For this review, take the finished solid that the model builds, in its own axes (mm). Face numbers are marked on the shaded views. A direction names the side the tool comes from. Round coordinates to 2 decimals unless told otherwise and drop trailing zeros. Loops run counter-clockwise (first coordinate to the right, second up) from the corner with the lowest first, then second, coordinate; pieces in that order, holes last.
1) Wall thickness on L1, parallel to Y at x = -10, z = 2.25; L2, parallel to X at y = 10, z = 3.45; L3, parallel to Z at x = 4.25, y = 9.5: over which ranges is each line inside the solid? List them lowest first.
2) Insertion check: pin 1 (4 mm diameter, centred on x = 6.5, y = 10, fed in from +Z); pin 2 (1 mm diameter, centred on x = 4.5, z = 19, fed in from -Y). Each pin has a flat end and moves straight along its axis. Give the tip position at first contact, or say it passes through.
3) Take a section at D-D (z = 3.5). State the section outline as (x, y) points, then the cut area to 3 significant figures.
4) Take a section at B-B (x = -10). State the section outline as (y, z) points.
5) Tool access review of the marked faces 1 and 2: name each direction out of +Z, -Z, +X, -X, +Y, -Y from which nothing blocks a thin tool from reaching the whole face with its end or side.
6) Take a section at A-A (z = 35). State the section outline as (x, y) points, then the cut area to 3 significant figures.
7) Take a section at C-C (y = -10). State the section outline as (x, z) points.
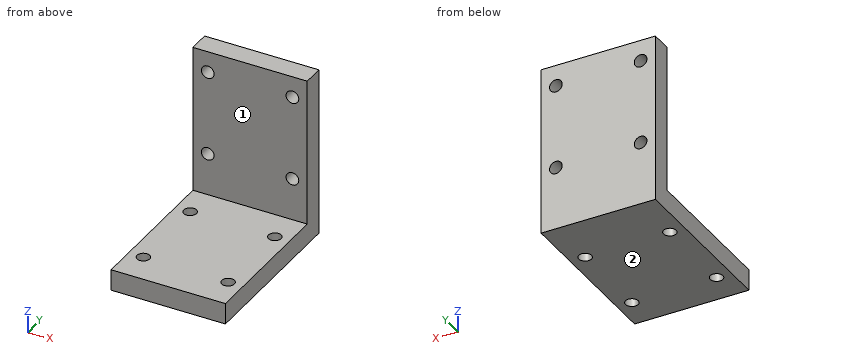
```python
from build123d import *

# Parameters (mm, degrees)
F0_W      = 27
F0_H      = 35
F1_DEPTH  = 5
F2_D      = 3
F1_FACE_W = 27
F1_FACE_H = 5
F3_DEPTH  = 5
F4_W      = 5
F4_H      = 40
F5_DEPTH  = 13.5
F7_D      = 3


with BuildPart() as f1:
    # F0 (on Top) → F1 (new body)
    with BuildSketch(Plane.XY):
        Rectangle(F0_W, F0_H)
    extrude(amount=F1_DEPTH)

    # F2 (through all)
    with Locations(Plane(origin=(0, 0, 0), x_dir=(1, 0, 0), z_dir=(0, 0, -1))):
        with Locations((-10, 10), (10, 10), (10, -10), (-10, -10)):
            Hole(F2_D / 2)

    # F1_face (on face) → F3 (join)
    with BuildSketch(Plane(origin=(0, 17.5, 2.5), x_dir=(-1, 0, 0), z_dir=(0, 1, 0))):
        Rectangle(F1_FACE_W, F1_FACE_H)
    extrude(amount=F3_DEPTH)

    # F4 (on Right) → F5 (join, symmetric)
    with BuildSketch(Plane.YZ):
        with Locations((20.017813, 20)):
            Rectangle(F4_W, F4_H)
    extrude(amount=F5_DEPTH, both=True)

    # F7 (through all)
    with Locations(Plane.XZ):
        with Locations((-10, 35), (10, 35), (10, 15), (-10, 15)):
            Hole(F7_D / 2)


solid = f1.part
```
Response:
1. L1: y = -17.5 to -11.5, -8.5 to 8.5, 11.5 to 22.52
1. L2: x = -13.5 to -11.5, -8.5 to 8.5, 11.5 to 13.5
1. L3: z = 0 to 5
2. pin 1: stops at z = 5
2. pin 2: stops at y = 17.52
3. outline: (-13.5, -17.5) - (13.5, -17.5) - (13.5, 22.52) - (-13.5, 22.52) - close; hole circle Ø3 at (-10, -10); hole circle Ø3 at (-10, 10); hole circle Ø3 at (10, -10); hole circle Ø3 at (10, 10)
3. area: 1,050 mm2
4. outline: (-17.5, 0) - (-11.5, 0) - (-11.5, 5) - (-17.5, 5) - close; (-8.5, 0) - (8.5, 0) - (8.5, 5) - (-8.5, 5) - close; (11.5, 0) - (22.52, 0) - (22.52, 13.5) - (17.52, 13.5) - (17.52, 5) - (11.5, 5) - close; (17.52, 16.5) - (22.52, 16.5) - (22.52, 33.5) - (17.52, 33.5) - close; (17.52, 36.5) - (22.52, 36.5) - (22.52, 40) - (17.52, 40) - close
5. face 1: +Z, +X, -X, -Y
5. face 2: -Z, +X, -X, +Y, -Y
6. outline: (-13.5, 17.52) - (-11.5, 17.52) - (-11.5, 22.52) - (-13.5, 22.52) - close; (-8.5, 17.52) - (8.5, 17.52) - (8.5, 22.52) - (-8.5, 22.52) - close; (11.5, 17.52) - (13.5, 17.52) - (13.5, 22.52) - (11.5, 22.52) - close
6. area: 105 mm2
7. outline: (-13.5, 0) - (-11.5, 0) - (-11.5, 5) - (-13.5, 5) - close; (-8.5, 0) - (8.5, 0) - (8.5, 5) - (-8.5, 5) - close; (11.5, 0) - (13.5, 0) - (13.5, 5) - (11.5, 5) - close
